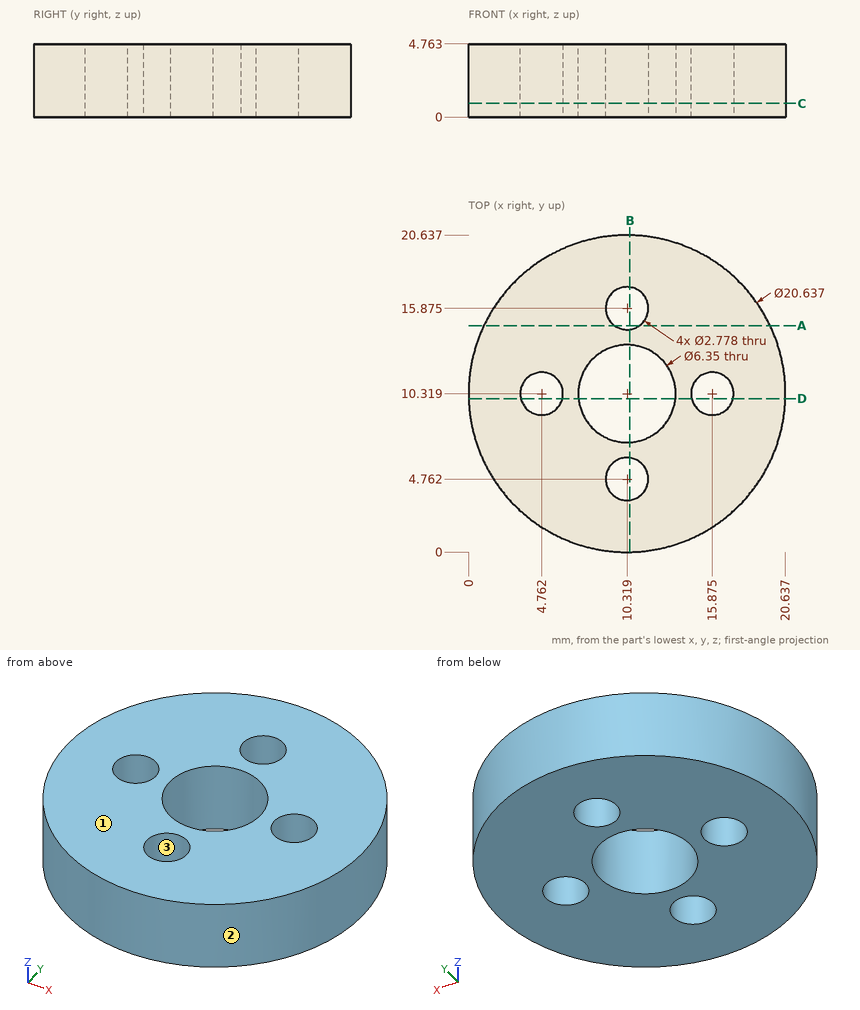
The drawing under review shows one solid part. Ordinate dimensions are in mm from its lowest x, y, z. Round coordinates to 2 decimals unless told otherwise and drop trailing zeros. Loops run counter-clockwise (first coordinate to the right, second up) from the corner with the lowest first, then second, coordinate; pieces in that order, holes last. Notation, with made-up numbers: (-23.5, 14.5) - (14.5, 14.5) arc R18 cw to (14.5, 38.5) - close; hole circle Ø11 at (-38.5, 17.5). An arc over 180 degrees is marked (long way). Put each result on its own line as item: value. Start each with the question number.
1. Consider section A-A on y = 14.75. State the section outline as (x, z) points.
2. Consider section B-B on x = 10.5. State the section outline as (y, z) points (1 decimal).
3. Insertion check: P1, Ø1.5, axis at y = 10, z = 1, coming from the +X side; P2, Ø1.5, axis at y = 11.5, z = 2, coming from the -X side; P3, Ø1.7, axis at x = 15.88, y = 10.32, coming from the +Z side. Each pin has a flat end and moves straight along its axis. Give the tip position at first contact, or say it passes through.
4. Mouldability with a two-part tool opening along Y and no side actions: class the marked faces 1, 2 and 3 as +Y half, -Y half, draft (parallel to the pull), parting line (faces both ways), or undercut.
5. Consider section C-C on z = 0.9. State how many separate pieces and enclosed holes the cut face has.
6. Consider section D-D on y = 10. State the section outline as (x, z) points (1 decimal).
7. For probe 1 along X at (y, z) = (10.75, 3.7) (1 decimal); probe 2 along X at (y, z) = (10, 2.8) (1 decimal); probe 3 along Y at (x, z) = (11.5, 3.85) (1 decimal), list the stretches that pass through material, from the lowest coordinate up. Write a range as [from, to].
Result sheet:
1. outline: (1, 0) - (9.5, 0) - (9.5, 4.76) - (1, 4.76) - close; (11.13, 0) - (19.64, 0) - (19.64, 4.76) - (11.13, 4.76) - close
2. outline: (0, 0) - (3.4, 0) - (3.4, 4.8) - (0, 4.8) - close; (6.1, 0) - (7.1, 0) - (7.1, 4.8) - (6.1, 4.8) - close; (13.5, 0) - (14.5, 0) - (14.5, 4.8) - (13.5, 4.8) - close; (17.3, 0) - (20.6, 0) - (20.6, 4.8) - (17.3, 4.8) - close
3. P1: x = 20.64
3. P2: x = 0.01
3. P3: through
4. face 1: draft
4. face 2: parting line
4. face 3: undercut
5. separate pieces: 1
5. enclosed holes: 5
6. outline: (0, 0) - (3.4, 0) - (3.4, 4.8) - (0, 4.8) - close; (6.1, 0) - (7.2, 0) - (7.2, 4.8) - (6.1, 4.8) - close; (13.5, 0) - (14.5, 0) - (14.5, 4.8) - (13.5, 4.8) - close; (17.2, 0) - (20.6, 0) - (20.6, 4.8) - (17.2, 4.8) - close
7. probe 1: [0, 3.4], [6.1, 7.2], [13.5, 14.6], [17.2, 20.6]
7. probe 2: [0, 3.4], [6.1, 7.2], [13.5, 14.5], [17.2, 20.6]
7. probe 3: [0.1, 4], [5.5, 7.4], [13.3, 15.1], [16.6, 20.6]
